For this review, take the finished solid that the model builds, in its own axes (mm). A direction names the side the tool comes from. Round coordinates to 2 decimals unless told otherwise and drop trailing zeros. Write each loop counter-clockwise with the first axis right and the second up, starting at its lowest first coordinate (ties: lowest second). Pieces come first, ordered by that corner, then holes. Notation, with made-up numbers: M 19.25,38 L 68.25,38 A22 cw 68.25,71 Z; hole C 68,-20.75 d5. An arc over 180 degrees is marked long. One line per question, with ' | ' between items.
```python
from build123d import *

# Parameters (mm, degrees)
SKETCH4_W             = 31.4
SKETCH4_H             = 31.4
SKETCH4_W_2           = 25.4
SKETCH4_H_2           = 25.4
BOSS_EXTRUDE3_DEPTH   = 30
SKETCH5_W             = 31.4
SKETCH5_H             = 31.4
BOSS_EXTRUDE4_DEPTH   = 5
SKETCH6_W             = 31.4
SKETCH6_H             = 8
BOSS_EXTRUDE5_DEPTH   = 5
BOSS_EXTRUDE6_DEPTH   = 8
SKETCH8_R             = 9.5
BOSS_EXTRUDE7_DEPTH   = 8
SKETCH9_W             = 31.4
SKETCH9_H             = 10
BOSS_EXTRUDE8_DEPTH   = 5
SKETCH10_W            = 31.4
SKETCH10_H            = 10
BOSS_EXTRUDE9_DEPTH   = 13
SKETCH11_W            = 6.2
SKETCH11_H            = 10
BOSS_EXTRUDE10_DEPTH  = 40
BOSS_EXTRUDE11_DEPTH  = 3
SKETCH13_W            = 31.4
SKETCH13_H            = 31.4
CUT_EXTRUDE1_DEPTH    = 31.4
SKETCH14_W            = 31.4
SKETCH14_H            = 31.4
BOSS_EXTRUDE12_DEPTH  = 4
SKETCH16_W            = 31.4
SKETCH16_H            = 8
BOSS_EXTRUDE13_DEPTH  = 15.4
CUT_EXTRUDE3_START    = 8
SKETCH8_2_R           = 9.5
CUT_EXTRUDE3_DEPTH    = 24
MIRROR2_START         = -15.7
MIRROR2_DEPTH         = 36.4
MIRROR2_START_2       = 12.7
MIRROR2_2_OUTLINE_W   = 6.2
MIRROR2_2_OUTLINE_H   = 13
MIRROR2_2_DEPTH       = 48
MIRROR2_START_3       = -4
MIRROR2_3_OUTLINE_R   = 9.5
MIRROR2_3_DEPTH       = 8
MIRROR2_4_OUTLINE_W   = 31.4
MIRROR2_4_OUTLINE_H   = 10
MIRROR2_4_DEPTH       = 16
MIRROR2_5_OUTLINE_W   = 25.4
MIRROR2_5_OUTLINE_H   = 15.4
MIRROR2_5_DEPTH       = 8
MIRROR2_6_OUTLINE_W   = 25.4
MIRROR2_6_OUTLINE_H   = 12
MIRROR2_6_OUTLINE_W_2 = 19
MIRROR2_6_OUTLINE_H_2 = 5.4
MIRROR2_6_DEPTH       = 8
SKETCH17_W            = 30.8
SKETCH17_H            = 24
CUT_EXTRUDE2_DEPTH    = 31.4


# Read off the part's stored shape, not the designer's step: Mirror2
with BuildPart() as part:
    # Sketch4 → Boss-Extrude3 (new body)
    with BuildSketch(Plane.XY):
        Rectangle(SKETCH4_W, SKETCH4_H)
        Rectangle(SKETCH4_W_2, SKETCH4_H_2, mode=Mode.SUBTRACT)
    extrude(amount=BOSS_EXTRUDE3_DEPTH)

    # Sketch5 → Boss-Extrude4 (add)
    with BuildSketch(Plane.XY.offset(30)):
        Rectangle(SKETCH5_W, SKETCH5_H)
    extrude(amount=BOSS_EXTRUDE4_DEPTH)

    # Sketch6 → Boss-Extrude5 (add)
    with BuildSketch(Plane.XY.offset(35)):
        Rectangle(SKETCH6_W, SKETCH6_H)
    extrude(amount=BOSS_EXTRUDE5_DEPTH)

    # Sketch7 → Boss-Extrude6 (add)
    with BuildSketch(Plane.XZ.offset(4)):
        with BuildLine():
            Line((-15.7, 40), (-15.7, 52))
            ThreePointArc((-15.7, 52), (-11.306601718, 62.606601718), (-0.7, 67))
            Line((-0.7, 67), (0.7, 67))
            ThreePointArc((0.7, 67), (11.306601718, 62.606601718), (15.7, 52))
            Line((15.7, 52), (15.7, 40))
            Line((15.7, 40), (-15.7, 40))
        make_face()
    extrude(amount=-BOSS_EXTRUDE6_DEPTH)

    # Sketch8 → Boss-Extrude7 (add)
    with BuildSketch(Plane.XZ.offset(4)):
        with Locations(Location((0, 52, 0), (0, 0, 180))):
            Circle(SKETCH8_R)
    boss_extrude7 = extrude(amount=BOSS_EXTRUDE7_DEPTH)

    # Mirror1: Boss-Extrude7 across plane
    add(boss_extrude7.mirror(Plane.ZX))

    # Sketch9 → Boss-Extrude8 (add)
    with BuildSketch(Plane(origin=(0, 15.7, 0), x_dir=(1, 0, 0), z_dir=(0, 1, 0))):
        with Locations((0, -27)):
            Rectangle(SKETCH9_W, SKETCH9_H)
    extrude(amount=BOSS_EXTRUDE8_DEPTH)

    # Sketch10 → Boss-Extrude9 (add)
    with BuildSketch(Plane(origin=(0, 15.7, 0), x_dir=(1, 0, 0), z_dir=(0, 1, 0))):
        with Locations((0, -17)):
            Rectangle(SKETCH10_W, SKETCH10_H)
    extrude(amount=BOSS_EXTRUDE9_DEPTH)

    # Sketch11 → Boss-Extrude10 (add)
    with BuildSketch(Plane(origin=(0, 20.7, 0), x_dir=(1, 0, 0), z_dir=(0, 1, 0))):
        with Locations((-12.6, -27)):
            Rectangle(SKETCH11_W, SKETCH11_H)
        with Locations((12.6, -27)):
            Rectangle(SKETCH11_W, SKETCH11_H)
    extrude(amount=BOSS_EXTRUDE10_DEPTH)

    # Sketch12 → Boss-Extrude11 (add)
    with BuildSketch(Plane.XY.offset(32)):
        Polygon((-15.7, 60.7), (-9.5, 60.7), (-9.5, 20.7), (9.5, 20.7), (9.5, 60.7), (15.7, 60.7), (15.7, 15.7), (-15.7, 15.7), align=None)
    extrude(amount=BOSS_EXTRUDE11_DEPTH)

    # Sketch13 → Cut-Extrude1 (cut)
    with BuildSketch(Plane.ZY.offset(15.7)):
        with Locations((15.7, 0)):
            Rectangle(SKETCH13_W, SKETCH13_H)
    extrude(amount=-CUT_EXTRUDE1_DEPTH, mode=Mode.SUBTRACT)

    # Sketch14 → Boss-Extrude12 (add)
    with BuildSketch(Plane(origin=(0, 0, 31.4), x_dir=(-1, 0, 0), z_dir=(0, 0, -1))):
        Rectangle(SKETCH14_W, SKETCH14_H)
    extrude(amount=BOSS_EXTRUDE12_DEPTH)

    # Sketch16 → Boss-Extrude13 (add)
    with BuildSketch(Plane(origin=(0, 0, 27.4), x_dir=(-1, 0, 0), z_dir=(0, 0, -1))):
        with Locations((0, -11.7)):
            Rectangle(SKETCH16_W, SKETCH16_H)
    extrude(amount=BOSS_EXTRUDE13_DEPTH)

    # Sketch8<2> → Cut-Extrude3 (cut)
    with BuildSketch(Plane.XZ.offset(4).offset(CUT_EXTRUDE3_START)):
        with Locations(Location((0, 52, 0), (0, 0, 270))):
            Circle(SKETCH8_2_R)
    extrude(amount=-CUT_EXTRUDE3_DEPTH, mode=Mode.SUBTRACT)

    # Mirror2 outline → Mirror2 (add)
    with BuildSketch(Plane(origin=(0, 0, 0), x_dir=(1, 0, 0), z_dir=(0, 1, 0)).offset(MIRROR2_START)):
        Polygon((12.7, -24), (15.7, -24), (15.7, 11), (-15.7, 11), (-15.7, -24), (-12.7, -24), (-12.7, 3.4), (12.7, 3.4), align=None)
    extrude(amount=MIRROR2_DEPTH)

    # Mirror2 2 outline → Mirror2 2 (add)
    with BuildSketch(Plane(origin=(0, 0, 0), x_dir=(1, 0, 0), z_dir=(0, 1, 0)).offset(MIRROR2_START_2)):
        with Locations((12.6, 4.5)):
            Rectangle(MIRROR2_2_OUTLINE_W, MIRROR2_2_OUTLINE_H)
        with Locations((-12.6, 4.5)):
            Rectangle(MIRROR2_2_OUTLINE_W, MIRROR2_2_OUTLINE_H)
    extrude(amount=MIRROR2_2_DEPTH)

    # Mirror2 3 outline → Mirror2 3 (add)
    with BuildSketch(Plane(origin=(0, 0, 0), x_dir=(1, 0, 0), z_dir=(0, 1, 0)).offset(MIRROR2_START_3)):
        with BuildLine():
            Line((-15.7, 11), (15.7, 11))
            Line((15.7, 11), (15.7, 28))
            ThreePointArc((15.7, 28), (11.306601718, 38.606601718), (0.7, 43))
            Line((0.7, 43), (-0.7, 43))
            ThreePointArc((-0.7, 43), (-11.306601718, 38.606601718), (-15.7, 28))
            Line((-15.7, 28), (-15.7, 11))
        make_face()
        with Locations((0, 28)):
            Circle(MIRROR2_3_OUTLINE_R, mode=Mode.SUBTRACT)
    extrude(amount=MIRROR2_3_DEPTH)

    # Mirror2 4 outline → Mirror2 4 (add)
    with BuildSketch(Plane(origin=(0, 0, 0), x_dir=(1, 0, 0), z_dir=(0, 1, 0)).offset(MIRROR2_START_2)):
        with Locations((0, -7)):
            Rectangle(MIRROR2_4_OUTLINE_W, MIRROR2_4_OUTLINE_H)
    extrude(amount=MIRROR2_4_DEPTH)

    # Mirror2 5 outline → Mirror2 5 (add)
    with BuildSketch(Plane(origin=(0, 0, 0), x_dir=(1, 0, 0), z_dir=(0, 1, 0)).offset(MIRROR2_START)):
        with Locations((0, -4.3)):
            Rectangle(MIRROR2_5_OUTLINE_W, MIRROR2_5_OUTLINE_H)
    extrude(amount=MIRROR2_5_DEPTH)

    # Mirror2 6 outline → Mirror2 6 (add)
    with BuildSketch(Plane(origin=(0, 0, 0), x_dir=(1, 0, 0), z_dir=(0, 1, 0)).offset(MIRROR2_START_2)):
        with Locations((0, -18)):
            Rectangle(MIRROR2_6_OUTLINE_W, MIRROR2_6_OUTLINE_H)
        with Locations((0, 0.7)):
            Rectangle(MIRROR2_6_OUTLINE_W_2, MIRROR2_6_OUTLINE_H_2)
    extrude(amount=MIRROR2_6_DEPTH)

    # Sketch17 → Cut-Extrude2 (cut)
    with BuildSketch(Plane.ZY.offset(15.7)):
        with Locations((12, 3.7)):
            Rectangle(SKETCH17_W, SKETCH17_H)
    extrude(amount=-CUT_EXTRUDE2_DEPTH, mode=Mode.SUBTRACT)


solid = part.part
```
Item 1: Machinability: for faces 1 (the face through (9.5, 40, -4)), 2 (the face through (-7, -4, -20)), 3 (the face through (7, 4, 44)), 4 (the face through (7, -4, 44)), 5 (the face through (13, 44, 2)), which of the approach directions +Z, -Z, +X, -X, +Y, -Y give a long, thin tool a straight path to every point of the face, cutting with its end or side? Answer none if there is none.
Results:
face 1: -Z, +Y | face 2: -Z, +X, -X, -Y | face 3: +Z, +X, -X, +Y | face 4: +Z, +X, -X, -Y | face 5: +X, -X, +Y
Item 2: Take a section at A-A (z = 25). Write out the cut boundary in (x, y), then the cut area to 3 significant figures.
Results:
outline: M -15.7,-15.7 L 15.7,-15.7 L 15.7,-8.3 L -15.7,-8.3 Z; M -15.7,15.7 L 15.7,15.7 L 15.7,60.7 L 9.5,60.7 L 9.5,20.7 L -9.5,20.7 L -9.5,60.7 L -15.7,60.7 Z | area: 885 mm2
Item 3: To check wall thickness, follow line 1 along Y through (x, z) = (-11.5, 12.5); line 2 along X through (y, z) = (-2, -28); line 3 along Z through (x, y) = (4, -7). State the ranges of each line that lie inside material, in increasing order. Write a range as from..to.
Results:
line 1: -15.7..-8.3, 15.7..28.7 | line 2: -15.7..-9.5, 9.5..15.7 | line 3: -11..-3.4, 27.4..35
Item 4: Take a section at C-C (x = 2). Write out the cut boundary in (y, z), then the cut area to 3 significant figures.
Results:
outline: M -15.7,-11 L -4,-11 L -4,-18.71 L 4,-18.71 L 4,-11 L 20.7,-11 L 20.7,2 L 28.7,2 L 28.7,22 L 20.7,22 L 20.7,35 L 4,35 L 4,42.71 L -4,42.71 L -4,35 L -15.7,35 Z; M -4,-42.94 L 4,-42.94 L 4,-37.29 L -4,-37.29 Z; M -4,61.29 L 4,61.29 L 4,66.94 L -4,66.94 Z; hole M -8.3,-3.4 L 15.7,-3.4 L 15.7,27.4 L -8.3,27.4 Z | area: 1,310 mm2
Item 5: Mouldability with a two-part tool opening along Z and no side actions: class faces 6 (the face through (0, 4, 27.4)), 7 (the face through (-9.5, 41, 28)), 8 (the face through (0, 25, 2)) as +Z half, -Z half, draft (parallel to the pull), parting line (faces both ways), or undercut.
Results:
face 6: undercut | face 7: draft | face 8: -Z half
Item 6: Take a section at D-D (y = 23). Write out the cut boundary in (x, z).
Results:
outline: M -15.7,-11 L -9.5,-11 L -9.5,2 L 9.5,2 L 9.5,-11 L 15.7,-11 L 15.7,35 L 9.5,35 L 9.5,22 L -9.5,22 L -9.5,35 L -15.7,35 Z
Item 7: Take a section at B-B (y = 46). Write out the cut boundary in (x, z), then the cut area to 3 significant figures.
Results:
outline: M -15.7,-11 L -9.5,-11 L -9.5,2 L -15.7,2 Z; M -15.7,22 L -9.5,22 L -9.5,35 L -15.7,35 Z; M 9.5,-11 L 15.7,-11 L 15.7,2 L 9.5,2 Z; M 9.5,22 L 15.7,22 L 15.7,35 L 9.5,35 Z | area: 322 mm2
Item 8: Insertion check: pin 1 Ø3 at (x, y) = (-12.5, 39) entering from -Z; pin 2 Ø12 at (x, z) = (-6.5, 49.5) entering from +Y; pin 3 Ø3 at (x, y) = (-5.5, 26) entering from -Z. Each pin has a flat end and moves straight along its axis. Give the tip position at first contact, or say it passes through.
Results:
pin 1: z = -11 | pin 2: y = 4 | pin 3: z = 2
